Could you check a few things on this model? Use its own coordinates, in mm. Face numbers are marked on the shaded views. A direction names the side the tool comes from. Give positions to 0.01 mm unless a question says otherwise; leave off trailing zeros. Write each loop counter-clockwise with the first axis right and the second up, starting at its lowest first coordinate (ties: lowest second). Pieces come first, ordered by that corner, then holes. Notation, with made-up numbers: (20, 63.25) - (77, 63.25) arc R14 ccw to (77, 77.25) - close; hole circle Ø11 at (14.5, 46.25). An arc over 180 degrees is marked (long way). Answer as CSV lines item,"result". Start each with the question number.
Q1. Will these pins go through, and if not, where does the flat tip stop? pin 1 Ø8 at (x, y) = (21, 3) entering from +Z; pin 2 Ø1.5 at (x, z) = (22.5, 3.5) entering from +Y.
Q2. If I drill on line 1 along X through (y, z) = (-4.25, 5); line 2 along X through (y, z) = (4.25, 3.75); line 3 along Z through (x, y) = (3.5, 7), over which ranges is the centre line in solid material (lowest first)?
Q3. Imagine slicing it at D-D on z = 4.5. List the corners of the cut face in (x, y) for me.
Q4. On a 3-axis mill with a long thin cutter (end or side, diameter ignored), from which of +Z, -Z, +X, -X, +Y, -Y can I reach the whole of each face in a straight line? I mean the marked faces 1 and 2. Say none if no direction works.
Q5. Imagine slicing it at A-A on z = 0. List the corners of the cut face in (x, y) for me.
Q6. Imagine slicing it at C-C on x = 2.5. List the corners of the cut face in (y, z) for me, and give its area (3 significant figures).
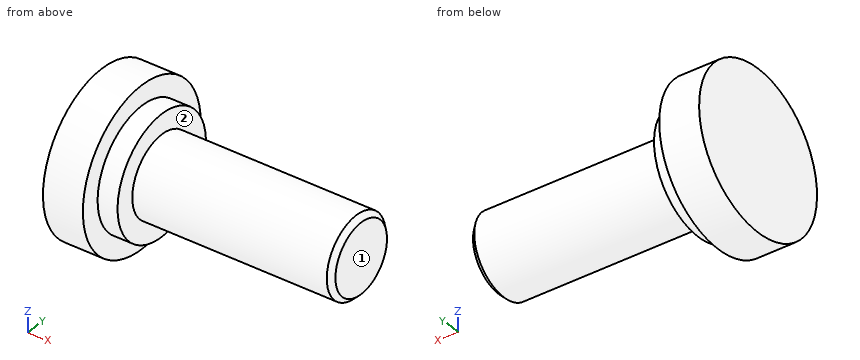
```python
from build123d import *

# Parameters (mm, degrees)
CHANFREIN1_SIZE = 0.5


with BuildPart() as part:
    # Esquisse1 → Base-Révolution (revolve)
    with BuildSketch(Plane.XY, mode=Mode.PRIVATE) as base_r_volution_sk:
        Polygon((0, 0), (0, 8), (4, 8), (4, 6), (6, 6), (6, 4), (26, 4), (26, 0), align=None)
    revolve(base_r_volution_sk.sketch.rotate(Axis((-4.18019429, 0, 0), (1, 0, 0)), 90), axis=Axis((-4.18019429, 0, 0), (1, 0, 0)))

    # Chanfrein1
    chanfrein1_edges = [part.edges().sort_by_distance(p)[0] for p in [
        (26, 0, -4),
    ]]
    chamfer(chanfrein1_edges, length=CHANFREIN1_SIZE)


solid = part.part
```
Conclusion:
1,pin 1,"z = 4"
1,pin 2,"y = 2.9"
2,line 1,"0 to 4"
2,line 2,"0 to 6"
2,line 3,"-3.87 to 3.87"
3,outline,"(0, -6.61) - (4, -6.61) - (4, -3.97) - (6, -3.97) - (6, 3.97) - (4, 3.97) - (4, 6.61) - (0, 6.61) - close"
4,face 1,"+Z, -Z, +X, +Y, -Y"
4,face 2,"+X"
5,outline,"(0, -8) - (4, -8) - (4, -6) - (6, -6) - (6, -4) - (25.5, -4) - (26, -3.5) - (26, 3.5) - (25.5, 4) - (6, 4) - (6, 6) - (4, 6) - (4, 8) - (0, 8) - close"
6,outline,"circle Ø16 at (0, 0)"
6,area,"201 mm^2"
